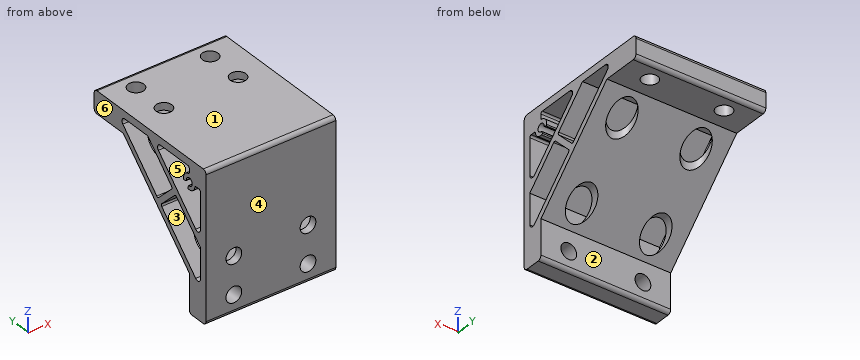
from build123d import *

# Parameters (mm, degrees)
BOSS_EXTRUDE1_DEPTH = 35
DIAMETERHOLE1_D     = 8.5
DIAMETERHOLE1_DEPTH = 12
DIAMETERHOLE2_D     = 8.5
DIAMETERHOLE2_DEPTH = 12.001
DIAMETERHOLE3_REACH = 120.427
SKETCH6_R           = 7
DIAMETERHOLE4_REACH = 120.427
SKETCH7_R           = 7
LPATTERN1_COUNT     = 2
LPATTERN1_PITCH     = 40


with BuildPart() as part:
    # Sketch1 → Boss-Extrude1 (new, symmetric)
    with BuildSketch(Plane(origin=(0, 0, 0), x_dir=(0, 0, -1), z_dir=(1, 0, 0))):
        with BuildLine():
            Line((2, 0), (78, 0))
            ThreePointArc((78, 0), (79.414213562, 0.585786438), (80, 2))
            Line((80, 2), (80, 10))
            ThreePointArc((80, 10), (79.414213562, 11.414213562), (78, 12))
            Line((78, 12), (59.176911935, 12))
            Line((59.176911935, 12), (12, 59.176911935))
            Line((12, 59.176911935), (12, 78))
            ThreePointArc((12, 78), (11.414213562, 79.414213562), (10, 80))
            Line((10, 80), (2, 80))
            ThreePointArc((2, 80), (0.585786438, 79.414213562), (0, 78))
            Line((0, 78), (0, 2))
            ThreePointArc((0, 2), (0.585786438, 0.585786438), (2, 0))
        make_face()
        with BuildLine():
            Line((7.414213562, 34.064213562), (34.064213562, 7.414213562))
            ThreePointArc((34.064213562, 7.414213562), (34.497759065, 5.234633135), (32.65, 4))
            Line((32.65, 4), (13, 4))
            ThreePointArc((13, 4), (12.292893219, 4.292893219), (12, 5))
            Line((12, 5), (12, 7.427254654))
            ThreePointArc((12, 7.427254654), (12.127727309, 7.761040579), (12.445652174, 7.924292192))
            ThreePointArc((12.445652174, 7.924292192), (15.214400117, 9.454880771), (16.069295651, 12.500832214))
            ThreePointArc((16.069295651, 12.500832214), (15.852577049, 12.854314019), (15.443630561, 12.922718028))
            Line((15.443630561, 12.922718028), (14.464530927, 12.660369072))
            ThreePointArc((14.464530927, 12.660369072), (14.187104489, 12.468068335), (14.095105748, 12.143289589))
            ThreePointArc((14.095105748, 12.143289589), (10.51507576, 10.51507576), (12.143289589, 14.095105748))
            ThreePointArc((12.143289589, 14.095105748), (12.468068335, 14.187104489), (12.660369072, 14.464530927))
            Line((12.660369072, 14.464530927), (12.922718028, 15.443630561))
            ThreePointArc((12.922718028, 15.443630561), (12.854314019, 15.852577049), (12.500832214, 16.069295651))
            ThreePointArc((12.500832214, 16.069295651), (9.454880771, 15.214400117), (7.924292192, 12.445652174))
            ThreePointArc((7.924292192, 12.445652174), (7.761040579, 12.127727309), (7.427254654, 12))
            Line((7.427254654, 12), (5, 12))
            ThreePointArc((5, 12), (4.292893219, 12.292893219), (4, 13))
            Line((4, 13), (4, 32.65))
            ThreePointArc((4, 32.65), (5.234633135, 34.497759065), (7.414213562, 34.064213562))
        make_face(mode=Mode.SUBTRACT)
        with BuildLine():
            Line((4, 58.105844123), (4, 41.721067812))
            Line((4, 41.721067812), (21.092766953, 24.628300859))
            ThreePointArc((21.092766953, 24.628300859), (21.799873734, 24.33540764), (22.506980515, 24.628300859))
            Line((22.506980515, 24.628300859), (31.699368671, 33.820689014))
            ThreePointArc((31.699368671, 33.820689014), (31.99226189, 34.527795796), (31.699368671, 35.234902577))
            Line((31.699368671, 35.234902577), (7.414213562, 59.520057685))
            ThreePointArc((7.414213562, 59.520057685), (5.234633135, 59.953603188), (4, 58.105844123))
        make_face(mode=Mode.SUBTRACT)
        with BuildLine():
            Line((33.820689014, 31.699368671), (24.628300859, 22.506980515))
            ThreePointArc((24.628300859, 22.506980515), (24.33540764, 21.799873734), (24.628300859, 21.092766953))
            Line((24.628300859, 21.092766953), (41.721067812, 4))
            Line((41.721067812, 4), (58.105844123, 4))
            ThreePointArc((58.105844123, 4), (59.953603188, 5.234633135), (59.520057685, 7.414213562))
            Line((59.520057685, 7.414213562), (35.234902577, 31.699368671))
            ThreePointArc((35.234902577, 31.699368671), (34.527795796, 31.99226189), (33.820689014, 31.699368671))
        make_face(mode=Mode.SUBTRACT)
    extrude(amount=BOSS_EXTRUDE1_DEPTH, both=True)

    # DiameterHole1
    with Locations(Plane.XY):
        with Locations((-20, 70), (-20, 50)):
            diameterhole1 = Hole(DIAMETERHOLE1_D / 2, depth=DIAMETERHOLE1_DEPTH)

    # DiameterHole2
    with Locations(Plane(origin=(0, 0, 0), x_dir=(-1, 0, 0), z_dir=(0, -1, 0))):
        with Locations((20, 70), (20, 50)):
            diameterhole2 = Hole(DIAMETERHOLE2_D / 2, depth=DIAMETERHOLE2_DEPTH)

    # DiameterHole3: up to this plane
    diameterhole3_end = Plane(origin=(35, 7.414213562, -59.520057685), z_dir=(0, -0.7071067811865515, 0.7071067811865437))
    # Sketch6 → DiameterHole3 (cut, up to the surface)
    with BuildSketch(Plane(origin=(0, 80, 0), x_dir=(1, 0, 0), z_dir=(0, 1, 0)), mode=Mode.PRIVATE) as diameterhole3_sk1:
        with Locations(Location((-20, 50, 0), (0, 0, 270))):
            Circle(SKETCH6_R)
    diameterhole3_tool1 = split(extrude(diameterhole3_sk1.sketch, amount=-DIAMETERHOLE3_REACH, mode=Mode.PRIVATE), bisect_by=diameterhole3_end, keep=Keep.BOTH, mode=Mode.PRIVATE)
    diameterhole3 = diameterhole3_tool1.solids().sort_by_distance((-20, 80, -50))[0]
    add(diameterhole3, mode=Mode.SUBTRACT)

    # DiameterHole4: up to this plane
    diameterhole4_end = Plane(origin=(35, 35.234902577, -31.699368671), z_dir=(0, -0.7071067811865511, 0.707106781186544))
    # Sketch7 → DiameterHole4 (cut, up to the surface)
    with BuildSketch(Plane(origin=(0, 0, -80), x_dir=(-1, 0, 0), z_dir=(0, 0, -1)), mode=Mode.PRIVATE) as diameterhole4_sk1:
        with Locations(Location((20, 50, 0), (0, 0, 270))):
            Circle(SKETCH7_R)
    diameterhole4_tool1 = split(extrude(diameterhole4_sk1.sketch, amount=-DIAMETERHOLE4_REACH, mode=Mode.PRIVATE), bisect_by=diameterhole4_end, keep=Keep.BOTH, mode=Mode.PRIVATE)
    diameterhole4 = diameterhole4_tool1.solids().sort_by_distance((-20, 50, -80))[0]
    add(diameterhole4, mode=Mode.SUBTRACT)

    # LPattern1: DiameterHole1, DiameterHole2, DiameterHole3, DiameterHole4 ×2
    with Locations(*[(i * LPATTERN1_PITCH, 0, 0) for i in range(1, LPATTERN1_COUNT)]):
        add(diameterhole1, mode=Mode.SUBTRACT)
        add(diameterhole2, mode=Mode.SUBTRACT)
        add(diameterhole3, mode=Mode.SUBTRACT)
        add(diameterhole4, mode=Mode.SUBTRACT)


solid = part.part
Source: CAD feature listing. Evaluate the final solid. Frame: model axes, mm. Face numbers are marked on the shaded views. A direction names the side the tool comes from. Coordinates: 2 decimals unless noted, no trailing zeros. Loops run counter-clockwise (first coordinate to the right, second up) from the corner with the lowest first, then second, coordinate; pieces in that order, holes last. Notation, with made-up numbers: (84, -14.75) - (128, -14.75) arc R20 ccw to (128, 11.25) - close; hole circle Ø10 at (23.5, -11). An arc over 180 degrees is marked (long way). One line per question, with ' | ' between items.
1) Pull-direction query (Y, two-part tool) for the marked faces 4, 5 and 6; classes: released by +Y, released by -Y, zero draft, split by the parting line, or undercut.
Report:
face 4: released by -Y | face 5: undercut | face 6: zero draft
2) First-contact query: P1, Ø2, axis at x = 14.5, z = -15.5, coming from the +Y side; P2, Ø11, axis at x = 20, z = -50, coming from the +Y side; P3, Ø9.5, axis at x = -15, z = -68, coming from the +Y side; P4, Ø5, axis at x = 20, y = 70, coming from the -Z side. Flat tips, straight axial feed; report the tip coordinate or a pass-through.
Report:
P1: stops at y = 56.68 | P2: stops at y = 4 | P3: stops at y = 12 | P4: passes through
3) Section D-D, the plane x = -20. Give the number of separate pieces and of enclosed holes in the cut face, then the cut area to 3 significant figures.
Report:
separate pieces: 5 | enclosed holes: 1 | area: 1,060 mm²
4) Set-up query: the marked faces 1, 2 and 3. Return all of +Z, -Z, +X, -X, +Y, -Y with unobstructed straight access to the full face (end or side cutting, diameter ignored); none if empty.
Report:
face 1: +Z, +X, -X, +Y, -Y | face 2: -Z, +X, -X, +Y | face 3: +X, -X
5) Line query: line 1 along Z through (x, y) = (20, 2); line 2 along X through (y, z) = (2.5, -70); line 3 along X through (y, z) = (50, -17). Output: solid intervals per line, ascending.
Report:
line 1: z = -80 to -74.25, -65.75 to -54.25, -45.75 to 0 | line 2: x = -35 to -24.25, -15.75 to 15.75, 24.25 to 35 | line 3: x = -35 to -27, -13 to 13, 27 to 35
6) Section A-A, the plane y = 70. Return loops of the section in (x, z).
Report:
outline: (-35, -12) - (-24.25, -12) - (-24.25, 0) - (-35, 0) - close; (-15.75, -12) - (15.75, -12) - (15.75, 0) - (-15.75, 0) - close; (24.25, -12) - (35, -12) - (35, 0) - (24.25, 0) - close
7) Section B-B, the plane z = -70. Return loops of the section in (x, y), then the cut area to 3 significant figures.
Report:
outline: (-35, 0) - (-24.25, 0) - (-24.25, 12) - (-35, 12) - close; (-15.75, 0) - (15.75, 0) - (15.75, 12) - (-15.75, 12) - close; (24.25, 0) - (35, 0) - (35, 12) - (24.25, 12) - close | area: 636 mm²
8) Section C-C, the plane y = 50. Return loops of the section in (x, z).
Report:
outline: (-35, -21.18) - (-27, -21.18) - (-27, -16.93) - (-35, -16.93) - close; (-35, -4) - (-24.25, -4) - (-24.25, 0) - (-35, 0) - close; (-15.75, -4) - (15.75, -4) - (15.75, 0) - (-15.75, 0) - close; (-13, -21.18) - (13, -21.18) - (13, -16.93) - (-13, -16.93) - close; (24.25, -4) - (35, -4) - (35, 0) - (24.25, 0) - close; (27, -21.18) - (35, -21.18) - (35, -16.93) - (27, -16.93) - close
